```python
from build123d import *

# Parameters (mm, degrees)
F0_R          = 1.625
F1_DEPTH      = 8
F3_R          = 1.05
F4_DEPTH      = 18.076
F4_DEPTH_BACK = 18.076


with BuildPart() as f1:
    # F0 (on Top) → F1 (new body)
    with BuildSketch(Plane.XY):
        with BuildLine():
            Line((14.5, -15), (18.075, -15))
            Line((18.075, -15), (18.075, 0))
            ThreePointArc((18.075, 0), (16.9619981016, -2.247150974), (14.5, -2.7236235056))
            Line((14.5, -2.7236235056), (14.5, -15))
        make_face()
        with BuildLine():
            ThreePointArc((14.5, -2.7236235056), (16.9619981016, -2.247150974), (18.075, 0))
            ThreePointArc((18.075, 0), (15.25, 2.825), (12.425, 0))
            ThreePointArc((12.425, 0), (12.6406969517, -1.0826645843), (13.2548496297, -2))
            ThreePointArc((13.2548496297, -2), (13.8305386996, -2.4424894302), (14.5, -2.7236235056))
        make_face()
        with Locations((15.25, 0)):
            Circle(F0_R, mode=Mode.SUBTRACT)
        with BuildLine():
            ThreePointArc((13.2548496297, -2), (12.6406969517, -1.0826645843), (12.425, 0))
            Line((12.425, 0), (0, 0))
            Line((0, 0), (-12.425, 0))
            ThreePointArc((-12.425, 0), (-12.6406969517, -1.0826645843), (-13.2548496297, -2))
            Line((-13.2548496297, -2), (0, -2))
            Line((0, -2), (13.2548496297, -2))
        make_face()
        with BuildLine():
            ThreePointArc((-13.2548496297, -2), (-12.6406969517, -1.0826645843), (-12.425, 0))
            ThreePointArc((-12.425, 0), (-15.25, 2.825), (-18.075, 0))
            ThreePointArc((-18.075, 0), (-16.9619981016, -2.247150974), (-14.5, -2.7236235056))
            ThreePointArc((-14.5, -2.7236235056), (-13.8305386996, -2.4424894302), (-13.2548496297, -2))
        make_face()
        with Locations((-15.25, 0)):
            Circle(F0_R, mode=Mode.SUBTRACT)
        with BuildLine():
            ThreePointArc((-14.5, -2.7236235056), (-16.9619981016, -2.247150974), (-18.075, 0))
            Line((-18.075, 0), (-18.075, -15))
            Line((-18.075, -15), (-14.5, -15))
            Line((-14.5, -15), (-14.5, -2.7236235056))
        make_face()
    extrude(amount=F1_DEPTH)

    # F3 (on Right) → F4 (cut, two sides)
    with BuildSketch(Plane.YZ) as f4_sk:
        with Locations((-12.5, 2.4)):
            Circle(F3_R)
        Polygon((-15, 8), (-15, 4.5), (-2, 8), align=None)
    extrude(amount=-F4_DEPTH, mode=Mode.SUBTRACT)
    extrude(f4_sk.sketch, amount=F4_DEPTH_BACK, mode=Mode.SUBTRACT)

    # F7 (on offset) → F8 (revolve, cut)
    with BuildSketch(Plane.XY.offset(1.85)):
        Polygon((14, -1.5), (0, -1.5), (-14, -1.5), (-14, -4.7194751813), (0, -4.7194751813), (14, -4.7194751813), align=None)
    revolve(axis=Axis((3.4951923881, -14, 1.85), (1, 0, 0)), mode=Mode.SUBTRACT)


solid = f1.part
```
For this review, take the finished solid that the model builds, in its own axes (mm). A direction names the side the tool comes from. Round coordinates to 2 decimals unless told otherwise and drop trailing zeros. Write each loop counter-clockwise with the first axis right and the second up, starting at its lowest first coordinate (ties: lowest second). Pieces come first, ordered by that corner, then holes. Notation, with made-up numbers: (-8, -26) -> (23, -26) arc R20 cw to (23, -14) -> close; hole circle Ø1 at (83.5, 55.5). An arc over 180 degrees is marked (long way). One line per question, with ' | ' between items. Start each with the question number.
1) Machinability: for faces 1 (the cylindrical face through (-0.196, -1.526, 2.656)), 2 (the flat face through (0, 0, 4)), 3 (the cylindrical face through (-14.279, -2.653, 4.833)), which of the approach directions +Z, -Z, +X, -X, +Y, -Y give a long, thin tool a straight path to every point of the face, cutting with its end or side? Answer none if there is none.
2) Wall thickness on line 1 along Y through (x, z) = (15.4, 2.4); line 2 along X through (y, z) = (-3.5, 4.75) (3 decimals); line 3 along X through (y, z) = (-0.5, 1.5) (3 decimals): over which ranges is each line inside the solid? List them lowest first.
3) Add section C-C (y = -12.5). Write out the cut boundary in (x, z) (3 decimals), and give its area (3 significant figures).
4) For pin 1 Ø2.5 at (x, z) = (1, 2.5) entering from +Y; pin 2 Ø1.3 at (x, z) = (1.5, 7) entering from -Y; pin 3 Ø2.5 at (x, y) = (15.25, 0) entering from +Z; pin 4 Ø3.5 at (x, y) = (-15.25, 0) entering from -Z, all flat-tipped, find the tip position at first contact; note any pin that passes through.
5) Add section D-D (z = 6). Write out the cut boundary in (x, y) (3 decimals).
6) Mouldability with a two-part tool opening along X and no side actions: class faces 4 (the flat face through (-18.075, -6, 3)), 5 (the flat face through (14, -2, 3)), 6 (the flat face through (-1, -1, 0)) as +X half, -X half, draft (parallel to the pull), parting line (faces both ways), or undercut.
7) Add section B-B (z = 2.4). Write out the cut boundary in (x, y) (3 decimals), and give its area (3 significant figures).
8) Add section A-A (x = -15.25). Write out the cut boundary in (y, z) (3 decimals), and give its area (3 significant figures).
Reported:
1) face 1: -Y | face 2: +Z, -Z, +Y | face 3: +Z, -Z, -Y
2) line 1: y = -15 to -13.55, -11.45 to -1.62, 1.62 to 2.82 | line 2: x = -18.075 to -14.5, 14.5 to 18.075 | line 3: x = -18.075 to -16.796, -13.704 to 13.704, 16.796 to 18.075
3) outline: (-18.075, 0) -> (-14.5, 0) -> (-14.5, 1.35) -> (-18.075, 1.35) -> close; (-18.075, 3.45) -> (-14.5, 3.45) -> (-14.5, 5.173) -> (-18.075, 5.173) -> close; (14.5, 0) -> (18.075, 0) -> (18.075, 1.35) -> (14.5, 1.35) -> close; (14.5, 3.45) -> (18.075, 3.45) -> (18.075, 5.173) -> (14.5, 5.173) -> close | area: 22.0 mm²
4) pin 1: stops at y = 0 | pin 2: stops at y = -2 | pin 3: passes through | pin 4: stops at z = 0
5) outline: (-18.075, -9.429) -> (-14.5, -9.429) -> (-14.5, -2.724) arc R2.825 ccw to (-14, -2.533) -> (-14, -2.209) -> (-13.489, -2.209) arc R2.825 ccw to (-13.255, -2) -> (13.255, -2) arc R2.825 ccw to (13.489, -2.209) -> (14, -2.209) -> (14, -2.533) arc R2.825 ccw to (14.5, -2.724) -> (14.5, -9.429) -> (18.075, -9.429) -> (18.075, 0) arc R2.825 ccw to (12.425, 0) -> (-12.425, 0) arc R2.825 ccw to (-18.075, 0) -> close; hole circle Ø3.25 at (-15.25, 0); hole circle Ø3.25 at (15.25, 0)
6) face 4: -X half | face 5: undercut | face 6: draft
7) outline: (-18.075, -15) -> (-14.5, -15) -> (-14.5, -13.55) -> (-18.075, -13.55) -> close; (-18.075, -11.45) -> (-14.5, -11.45) -> (-14.5, -2.724) arc R2.825 ccw to (-14, -2.533) -> (-14, -1.512) -> (14, -1.512) -> (14, -2.533) arc R2.825 ccw to (14.5, -2.724) -> (14.5, -11.45) -> (18.075, -11.45) -> (18.075, 0) arc R2.825 ccw to (12.425, 0) -> (-12.425, 0) arc R2.825 ccw to (-18.075, 0) -> close; (14.5, -15) -> (18.075, -15) -> (18.075, -13.55) -> (14.5, -13.55) -> close; hole circle Ø3.25 at (-15.25, 0); hole circle Ø3.25 at (15.25, 0) | area: 146 mm²
8) outline: (-15, 0) -> (-1.625, 0) -> (-1.625, 8) -> (-2, 8) -> (-15, 4.5) -> close; (1.625, 0) -> (2.825, 0) -> (2.825, 8) -> (1.625, 8) -> close; hole circle Ø2.1 at (-12.5, 2.4) | area: 90.4 mm²
